```python
from build123d import *

# Parameters (mm, degrees)
SKETCH_R     = 3
PAD_DEPTH    = 50.3
SKETCH001_R  = 2
PAD001_DEPTH = 2
SKETCH002_R  = 3
PAD002_DEPTH = 1
SKETCH003_R  = 2
PAD003_DEPTH = 2
SKETCH004_R  = 3
PAD004_DEPTH = 1


with BuildPart() as part:
    # Sketch → Pad (new body)
    with BuildSketch(Plane.YZ):
        Circle(SKETCH_R)
    extrude(amount=PAD_DEPTH)

    # Sketch001 (on Face3 of Pad) → Pad001 (join)
    with BuildSketch(Plane.YZ.offset(50.3)):
        Circle(SKETCH001_R)
    extrude(amount=PAD001_DEPTH)

    # Sketch002 (on Face5 of Pad001) → Pad002 (join)
    with BuildSketch(Plane.YZ.offset(52.3)):
        Circle(SKETCH002_R)
    extrude(amount=PAD002_DEPTH)

    # Sketch003 (on Face7 of Pad002) → Pad003 (join)
    with BuildSketch(Plane(origin=(0, 0, 0), x_dir=(0, 1, 0), z_dir=(-1, 0, 0))):
        Circle(SKETCH003_R)
    extrude(amount=PAD003_DEPTH)

    # Sketch004 (on Face9 of Pad003) → Pad004 (join)
    with BuildSketch(Plane(origin=(-2, 0, 0), x_dir=(0, 1, 0), z_dir=(-1, 0, 0))):
        Circle(SKETCH004_R)
    extrude(amount=PAD004_DEPTH)


solid = part.part
```
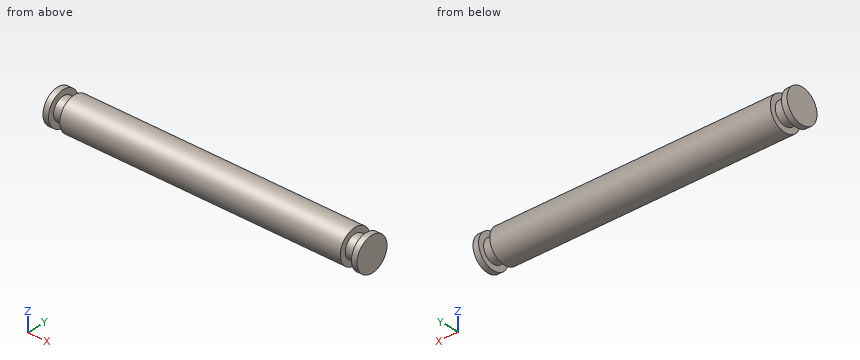
The model under review builds one solid part; all positions refer to its coordinate system, in mm. Round coordinates to 2 decimals unless told otherwise and drop trailing zeros. Write each loop counter-clockwise with the first axis right and the second up, starting at its lowest first coordinate (ties: lowest second). Pieces come first, ordered by that corner, then holes.
(1) We need section D-D on x = 48.5. Give the boundary of the cut face in (y, z).
(2) We need section A-A on y = -2.5. Give the boundary of the cut face in (x, z), and give its area (3 significant figures).
(3) Wall thickness on L1, parallel to X at y = 2.4, z = 1.75; L2, parallel to Z at x = 1, y = 0.1; L3, parallel to Y at x = 38, z = -0.2: over which ranges is each line inside the solid? List them lowest first.
(4) Insertion check: pin 1 (1 mm diameter, centred on x = 42.5, z = 1, fed in from +Y). The pin has a flat end and moves straight along its axis. Give the tip position at first contact, or say it passes through.
(5) We need section B-B on z = 0. Give the boundary of the cut face in (x, y).
Findings below:
1. outline: circle Ø6 at (0, 0)
2. outline: (-3, -1.66) - (-2, -1.66) - (-2, 1.66) - (-3, 1.66) - close; (0, -1.66) - (50.3, -1.66) - (50.3, 1.66) - (0, 1.66) - close; (52.3, -1.66) - (53.3, -1.66) - (53.3, 1.66) - (52.3, 1.66) - close
2. area: 173 mm2
3. L1: x = -3 to -2, 0 to 50.3, 52.3 to 53.3
3. L2: z = -3 to 3
3. L3: y = -2.99 to 2.99
4. pin 1: stops at y = 2.96
5. outline: (-3, -3) - (-2, -3) - (-2, -2) - (0, -2) - (0, -3) - (50.3, -3) - (50.3, -2) - (52.3, -2) - (52.3, -3) - (53.3, -3) - (53.3, 3) - (52.3, 3) - (52.3, 2) - (50.3, 2) - (50.3, 3) - (0, 3) - (0, 2) - (-2, 2) - (-2, 3) - (-3, 3) - close
